Autodesk Inventor part; units mm, degrees
ref_plane "Work Plane2" through (-67.5, -1, 0) normal (1, 0, 0) x (0, 0, -1)
ref_plane "Work Plane3" through (-76, 17.5, 0) normal (0, 1, 0) x (1, 0, 0)
ref_plane "YZ Plane" through (0, 0, 0) normal (1, 0, 0) x (0, 1, 0)
sketch "Sketch1" plane through (0, 0, 0) normal (0, 0, 1) x (1, 0, 0)
  line L0 (0, 0) -> (-75, 0)
  line L1 (-75, 0) -> (-75, 35)
  line L2 (-75, 35) -> (0, 35)
  line L3 (0, 35) -> (0, 0)
  line L4 (4, -4) -> (-79, -4)
  line L5 (-79, -4) -> (-79, 39)
  line L6 (-79, 39) -> (4, 39)
  line L7 (4, 39) -> (4, -4)
  line L8 (-37.5, 39) -> (-37.5, 56.2273) construction
  line L9 (-79, 17.5) -> (-92.6498, 17.5) construction
  line L10 (-65, 0) -> (-65, 35)
  line L11 (-35, 0) -> (-35, 35)
  circle A0 centre (-3, 32) radius 1
  circle A1 centre (-3, 3) radius 1
  line L12 (-3, 3) -> (-3, 32) construction
  line L13 (-3, 17.5) -> (-10.1857, 17.5) construction
  circle A2 centre (-75, 35) radius 0.5
  circle A3 centre (0, 35) radius 0.5
  circle A4 centre (-75, 0) radius 0.5
  circle A5 centre (0, 0) radius 0.5
  line L14 (-75.2, 35.2) -> (-75.2, -0.2)
  line L15 (-75.2, -0.2) -> (0.2, -0.2)
  line L16 (0.2, -0.2) -> (0.2, 35.2)
  line L17 (0.2, 35.2) -> (-75.2, 35.2)
  line L18 (-65, 0) -> (-65, -1.5)
  line L19 (-65, -1.5) -> (-35, -1.5)
  line L20 (-35, -1.5) -> (-35, 0)
  point P0 (-0.5, 35)
  point P1 (0, 34.5)
  point P2 (0, 0.5)
  point P3 (-0.5, 0)
  point P4 (-75, 0.5)
  point P5 (-74.5, 0)
  point P6 (-74.5, 35)
  point P7 (-75, 34.5)
  point P8 (0.2, 0.4583)
  point P9 (0.2, 34.5417)
  point P10 (-0.4583, 35.2)
  point P11 (-74.5417, 35.2)
  point P12 (-74.5417, -0.2)
  point P13 (-0.4583, -0.2)
  point P14 (-75.2, 34.5417)
  point P15 (-75.2, 0.4583)
  point P16 (-35, -0.2)
  point P17 (-65, -0.2)
  dimension "d0" = 75
  dimension "d1" = 35
  dimension "d2" = 4
  dimension "d8" = 10
  dimension "d9" = 40
  dimension "d10" = 2
  dimension "d11" = 2
  dimension "d12" = 29
  dimension "d13" = 3
  dimension "d18" = 1
  dimension "d21" = 75
  dimension "d24" = 35
  dimension "d32" = 0.2
  dimension "d33" = 1.5
extrude "Extrusion1" add sketch "Sketch1" along normal blind 4.6 contours L20 L15 L18 L0 | L11 L2 A3 L3 A5 L0 | L0 L10 L2 L11 | L0 A5 L15 L20 | L18 L15 A4 L0 | L0 A4 L1 A2 L2 L10 | A5 L3 L0 | L0 L3 A5 L16 L15 | L2 A2 L17 A3 | L20 L19 L18 L15 | A4 L15 L14 L1 L0 | L0 L1 A4 | L3 A3 L16 A5 | L15 L16 A5 | A3 L17 L16 L3 L2 | L2 L3 A3 | A4 L14 A2 L1 | A4 L14 L15 | A2 L1 L2 | L2 L1 A2 L14 L17 | A3 L16 L17 | L17 L14 A2 | L4 L5 L6 L7 | A0 | A1
extrude "Extrusion2" cut sketch "Sketch1" against normal blind 1.6 from surface at 4.6 contours L20 L15 L18 L0 | L11 L2 A3 L3 A5 L0 | L0 L10 L2 L11 | L0 A5 L15 L20 | L18 L15 A4 L0 | L0 A4 L1 A2 L2 L10 | A5 L3 L0 | L0 L3 A5 L16 L15 | L2 A2 L17 A3 | L20 L19 L18 L15 | A4 L15 L14 L1 L0 | L0 L1 A4 | L3 A3 L16 A5 | L15 L16 A5 | A3 L17 L16 L3 L2 | L2 L3 A3 | A4 L14 A2 L1 | A4 L14 L15 | A2 L1 L2 | L2 L1 A2 L14 L17 | A3 L16 L17 | L17 L14 A2 | A0 | A1
extrude "Extrusion3" cut sketch "Sketch1" against normal blind 2 from surface at 3 contours L0 L10 L2 L11
extrude "Extrusion4" cut sketch "Sketch1" against normal blind 3 from surface at 3 contours A0 | A1
chamfer "Chamfer2" distance 1 angle 45 2 edges at (-65, -0.2, 3.8) (-35, -0.2, 3.8)
fillet "Fillet1" radius 3 4 edges at (4, 39, 2.3) (-79, 39, 2.3) (-79, -4, 2.3) (4, -4, 2.3)
ref_plane "Work Plane1" through (-37.5, -1, 0) normal (1, 0, 0) x (0, 0, -1)
sketch "Sketch2" plane through (-37.5, -1, 0) normal (1, 0, 0) x (0, 0, -1)
  line L0 (-1, 1) -> (-3, 1)
  line L1 (-3, 1) -> (-4.6, 1)
  line L2 (-4.6, -3) -> (-4.6, 0)
  line L3 (-4.6, -0.8) -> (-4.6, 0.8)
  line L4 (-9.6, 0.8) -> (-9.6, -0.8)
  line L5 (-9.6, -0.8) -> (-4.6, -0.8)
  line L6 (-9.6, -0.8) -> (-9.6, -1.25)
  line L7 (-9.6, -1.25) -> (-8.6, -1.25)
  line L8 (-8.6, -1.25) -> (-8.15, -0.8)
  line L9 (-9.6, -0.8) -> (-9.15, -1.25)
  line L10 (-9.6, 0.8) -> (-4.6, 0.8)
  line L11 (-3, 0.8) -> (-4.6, 0.8)
  point P0 (0, 1)
  point P1 (-4.6, 1)
  point P2 (-4.6, -0.2)
  dimension "d41" = 1.6
  dimension "d42" = 0.45
  dimension "d45" = 45
  dimension "d46" = 45
  dimension "d47" = 1
  dimension "d51" = 5
ref_plane "Work Plane2" through (-67.5, -1, 0) normal (1, 0, 0) x (0, 0, -1)
extrude "Extrusion5" add sketch "Sketch2" against normal blind 32.5 and the other way blind 3.5 contours L5 L4 L10 L3 L2 | L8 L7 L9 L5
ref_plane "Work Plane3" through (-76, 17.5, 0) normal (0, 1, 0) x (1, 0, 0)
mirror "Mirror1" about plane through (-37.5, -1, 0) normal (1, 0, 0) of "Extrusion5"
fillet "Fillet4" radius 0.8 3 edges at (-37.5, -1.8, 4.6) (-5, -1, 4.6) (-70, -1, 4.6)
mirror "Mirror2" about plane through (-76, 17.5, 0) normal (0, 1, 0) of "Extrusion5", "Mirror1", "Fillet4"
sketch "Sketch7" plane through (0, 0, 4.6) normal (0, 0, 1) x (1, 0, 0)
  line L0 (-66, -0.2) -> (-66, -4)
  line L1 (-66, -4) -> (-34, -4)
  line L2 (-76, -4) -> (1, -4)
  line L3 (-34, -0.2) -> (-35, -1.2)
  line L4 (-34, -0.2) -> (-34, -4)
  line L5 (-66, -0.2) -> (-34, -0.2)
  point P0 (0, 0)
extrude "Extrusion10" cut sketch "Sketch7" along normal through all
fillet "Fillet5" radius 0.8 2 edges at (-66, -1.4, 4.6) (-34, -1.4, 4.6)
sketch "Sketch3" plane through (4, -1, 4.6) normal (1, 0, 0) x (0, 0, -1)
  line L0 (-8.3163, -11.6343) -> (11.7066, -11.6343)
  line L1 (11.7066, -11.6343) -> (11.7066, 46.4717)
  line L2 (11.7066, 46.4717) -> (-8.3163, 46.4717)
  line L3 (-8.3163, 46.4717) -> (-8.3163, -11.6343)
  point P0 (4.6, 1)
sketch "Sketch4" plane through (-74.5417, 35.2, 3) normal (0, 0, 1) x (1, 0, 0)
  line L0 (-6.3289, -41.6688) -> (13.4056, -41.6688)
  line L1 (13.4056, -41.6688) -> (13.4056, 7.8526)
  line L2 (13.4056, 7.8526) -> (-6.3289, 7.8526)
  line L3 (-6.3289, 7.8526) -> (-6.3289, -41.6688)
  point P0 (74.5417, -35.2)
sketch "Sketch5" plane through (-74.5417, 35.2, 4.6) normal (0, 0, -1) x (-1, 0, 0)
  line L0 (-3.0733, -37.6) -> (-8.5102, -37.6)
  line L1 (-3.6554, 1.6179) -> (-3.0733, 2.2)
  line L2 (-8.5102, -37.6) -> (-3.0733, -37.6)
  line L3 (-3.0733, -37.6) -> (-3.0733, 2.2)
  line L4 (-3.0733, 2.2) -> (-8.5102, 2.2)
  line L5 (-8.5102, 2.2) -> (-8.5102, -37.6)
  point P0 (-74.5417, -35.2)
sketch "Sketch6" plane through (-74.5417, 35.2, 4.6) normal (0, 0, 1) x (1, 0, 0)
  line L0 (3.0733, -37.6) -> (3.0733, 2.2)
  line L1 (8.5102, 2.2) -> (8.5102, -37.6)
  line L2 (3.0733, 0.0729) -> (8.5102, 0.0729)
  line L3 (8.5102, 0.0729) -> (8.5102, -35.4359)
  line L4 (8.5102, -35.4359) -> (3.0733, -35.4359)
  line L5 (3.0733, -35.4359) -> (3.0733, 0.0729)
  point P0 (74.5417, -35.2)
  point P1 (3.0733, -35.4359)
equation "\"d11\" = d10"
equation "\"d21\" = d0"
equation "\"d24\" = d1"
properties part number "scatola_v2_sotto"
Geometry check sheet. Reference: the model listing, model coordinates, mm. A direction names the side the tool comes from. Give positions to 0.01 mm unless a question says otherwise; leave off trailing zeros. Loops run counter-clockwise (first coordinate to the right, second up) from the corner with the lowest first, then second, coordinate; pieces in that order, holes last. Notation, with made-up numbers: M 70.5,65 L 80.5,65 A7 ccw 80.5,70 Z; hole C -9.5,47.5 d9. An arc over 180 degrees is marked long. Write item = value, one per line.
(1) Sectioned sample at A-A, the plane y = 32. Record the cut outline in (x, z), plus the area to 3 significant figures.
Answer below:
outline = M -79,0 L -4,0 L -4,3 L -35,3 L -35,1 L -65,1 L -65,3 L -75.2,3 L -75.2,4.6 L -79,4.6 Z; M -2,0 L 4,0 L 4,4.6 L 0.2,4.6 L 0.2,3 L -2,3 Z
area = 195 mm2
(2) Tool access check on faces 1 (the face through (-30, 17, 3)), 2 (the face through (-34, -1, 7)), 3 (the face through (-5, 36, 8)). Record the directions out of +Z, -Z, +X, -X, +Y, -Y that give a thin tool (end or side, any length) a straight path to the whole face; none if there is none.
Answer below:
face_1 = +Z
face_2 = +Z, -Y
face_3 = +Z, +X, +Y, -Y
(3) Sectioned sample at C-C, the plane x = -20.5. Record the cut outline in (y, z), plus the area to 3 significant figures.
Answer below:
outline = M -4,0 L 39,0 L 39,4.6 L 37.6,4.6 A0.8 cw 36.8,5.4 L 36.8,8.15 L 37.25,8.6 L 37.25,9.15 L 36.8,9.6 L 35.2,9.6 L 35.2,3 L -0.2,3 L -0.2,9.6 L -1.8,9.6 L -2.25,9.15 L -2.25,8.6 L -1.8,8.15 L -1.8,5.4 A0.8 cw -2.6,4.6 L -4,4.6 Z
area = 158 mm2
(4) Sectioned sample at D-D, the plane y = 6. Record the cut outline in (x, z), plus the area to 3 significant figures.
Answer below:
outline = M -79,0 L 4,0 L 4,4.6 L 0.2,4.6 L 0.2,3 L -35,3 L -35,1 L -65,1 L -65,3 L -75.2,3 L -75.2,4.6 L -79,4.6 Z
area = 201 mm2
(5) Release check for a two-part mould opening along X. For faces 4 (the face through (3.1, -3.14, 2.33)), 5 (the face through (-50, 18, 1)), 6 (the face through (-70, -1, 8)) record: released by +X, released by -X, zero draft, split by the parting line, or undercut.
Answer below:
face_4 = released by +X
face_5 = undercut
face_6 = released by -X
(6) Material ranges on line 1 (X direction, y = 13, z = 1.25); line 2 (Y direction, x = -39.5, z = 1.5); line 3 (Y direction, x = -27, z = 7.25), recorded low to high. Write a range as [from, to].
Answer below:
line_1 = [-79, -65], [-35, 4]
line_2 = [-4, 0], [35, 39]
line_3 = [-1.8, -0.2], [35.2, 36.8]
(7) Sectioned sample at B-B, the plane x = -3. Record the cut outline in (y, z), plus the area to 3 significant figures.
Answer below:
outline = M -4,0 L 2,0 L 2,3 L -0.2,3 L -0.2,4.6 L -4,4.6 Z; M 4,0 L 31,0 L 31,3 L 4,3 Z; M 33,0 L 39,0 L 39,4.6 L 35.2,4.6 L 35.2,3 L 33,3 Z
area = 129 mm2
(8) Gauge pin test, flat ends, axial feed: pin 1 Ø2 at (x, z) = (-42.5, 7.5) entering from +Y; pin 2 Ø1 at (y, z) = (-1.5, 7) entering from -X; pin 3 Ø1.4 at (x, z) = (-45.5, 6.5) entering from +Y. Record the tip position at first contact, or that the pin passes through.
Answer below:
pin_1 = 37.15
pin_2 = -70
pin_3 = 36.8
